```python
from build123d import *

# Parameters (mm, degrees)
BOSS_EXTRUDE1_DEPTH     = 32.5
SKETCH4_R               = 1.05
BOSS_EXTRUDE2_DEPTH     = 2.5
SKETCH5_R               = 1.05
BOSS_EXTRUDE3_DEPTH     = 3
CUT_EXTRUDE1_DEPTH      = 31.122
SKETCH13_W              = 30.122
SKETCH13_H              = 38
BOSS_EXTRUDE7_DEPTH     = 2.5
BOSS_EXTRUDE4_DEPTH     = 5
BOSS_EXTRUDE6_DEPTH     = 5
CUT_EXTRUDE2_DEPTH      = 6
SKETCH12_W              = 16.4999
SKETCH12_H              = 2
CUT_EXTRUDE4_DEPTH      = 10
CUT_EXTRUDE4_DEPTH_BACK = 23.5
CHAMFER1_SIZE           = 2
CHAMFER1_SIZE2          = 3.464101615


with BuildPart() as part:
    # Sketch2 → Boss-Extrude1 (new body)
    with BuildSketch(Plane(origin=(0, 0, 0), x_dir=(1, 0, 0), z_dir=(0, 1, 0))):
        Polygon((15.061, 0), (15.061, 32), (12.561, 32), (12.561, 2.5), (-12.561, 2.5), (-12.561, 32), (-15.061, 32), (-15.061, 0), align=None)
    extrude(amount=BOSS_EXTRUDE1_DEPTH)

    # Sketch4 → Boss-Extrude2 (add)
    with BuildSketch(Plane.XZ):
        Polygon((-7.5, -6), (7.5, -6), (12.561, -10), (15.061, -10), (15.061, 0), (-15.061, 0), (-15.061, -10), (-12.561, -10), align=None)
        with Locations((-10.2499, -4.95)):
            Circle(SKETCH4_R, mode=Mode.SUBTRACT)
        with Locations((10.2499, -4.95)):
            Circle(SKETCH4_R, mode=Mode.SUBTRACT)
    extrude(amount=BOSS_EXTRUDE2_DEPTH)

    # Sketch5 → Boss-Extrude3 (add)
    with BuildSketch(Plane(origin=(0, 32.5, 0), x_dir=(1, 0, 0), z_dir=(0, 1, 0))):
        Polygon((-15.061, 32), (-10.2499, 32), (-6.25, 26), (6.25, 26), (10.2499, 32), (15.061, 32), (15.061, 0), (-15.061, 0), align=None)
        with Locations((-10.2499, 8.7)):
            Circle(SKETCH5_R, mode=Mode.SUBTRACT)
        with Locations((10.2499, 8.7)):
            Circle(SKETCH5_R, mode=Mode.SUBTRACT)
    extrude(amount=BOSS_EXTRUDE3_DEPTH)

    # Sketch6 → Cut-Extrude1 (cut, through all)
    with BuildSketch(Plane.ZY.offset(15.061)):
        Polygon((-10, 0), (-32, 30.5), (-32, 0), align=None)
    extrude(amount=-CUT_EXTRUDE1_DEPTH, mode=Mode.SUBTRACT)

    # Sketch13 → Boss-Extrude7 (add)
    with BuildSketch(Plane.XY):
        with Locations((0, 16.5)):
            Rectangle(SKETCH13_W, SKETCH13_H)
    extrude(amount=BOSS_EXTRUDE7_DEPTH)

    # Sketch8 → Boss-Extrude4 (add)
    with BuildSketch(Plane.XY.offset(2.5)):
        Polygon((0, 76.5), (43.59255168, 16.5), (-43.59255168, 16.5), align=None)
    extrude(amount=BOSS_EXTRUDE4_DEPTH)

    # Sketch9 → Boss-Extrude6 (add)
    with BuildSketch(Plane.XY.offset(2.5)):
        Polygon((-43.59255168, 16.5), (-72.654252801, -23.5), (72.654252801, -23.5), (43.59255168, 16.5), align=None)
    extrude(amount=BOSS_EXTRUDE6_DEPTH)

    # Sketch10 → Cut-Extrude2 (cut, through all)
    with BuildSketch(Plane(origin=(0, 0, 2.5), x_dir=(-1, 0, 0), z_dir=(0, 0, -1))):
        Polygon((-43.59255168, -23.5), (-58.12340224, -3.5), (-72.654252801, -23.5), align=None)
        Polygon((72.654252801, -23.5), (58.12340224, -3.5), (43.59255168, -23.5), align=None)
    extrude(amount=-CUT_EXTRUDE2_DEPTH, mode=Mode.SUBTRACT)

    # Sketch12 → Cut-Extrude4 (cut, two sides)
    with BuildSketch(Plane(origin=(0, 0, -26), x_dir=(-1, 0, 0), z_dir=(0, 0, -1))) as cut_extrude4_sk:
        with Locations((0, 33.5)):
            Rectangle(SKETCH12_W, SKETCH12_H)
    extrude(amount=CUT_EXTRUDE4_DEPTH, mode=Mode.SUBTRACT)
    extrude(cut_extrude4_sk.sketch, amount=-CUT_EXTRUDE4_DEPTH_BACK, mode=Mode.SUBTRACT)

    # Chamfer1
    chamfer1_edges = [part.edges().sort_by_distance(p)[0] for p in [
        (-29.06170112, 36.5, 7.5),
        (0, -23.5, 7.5),
        (29.06170112, 36.5, 7.5),
        (50.85797696, -13.5, 7.5),
        (-50.85797696, -13.5, 7.5),
    ]]
    chamfer1_side = [part.faces().sort_by_distance(p)[0] for p in [
        (0, 12.152173913, 7.5),
    ]]
    chamfer(chamfer1_edges, length=CHAMFER1_SIZE, length2=CHAMFER1_SIZE2, reference=chamfer1_side[0])


solid = part.part
```
The model under review builds one solid part; all positions refer to its coordinate system, in mm. A direction names the side the tool comes from. Coordinates: 2 decimals unless noted, no trailing zeros. Write each loop counter-clockwise with the first axis right and the second up, starting at its lowest first coordinate (ties: lowest second). Pieces come first, ordered by that corner, then holes. Notation, with made-up numbers: (79.25, 39.25) - (130.25, 39.25) arc R23 cw to (130.25, 52.25) - close; hole circle Ø1 at (-28, 9.25). An arc over 180 degrees is marked (long way). Answer in a Markdown table with one row per item. Add a question column.
Q1. Consider section B-B on y = 11. Give the boundary of the cut face in (x, z).
Q2. Consider section C-C on z = -20. Give the boundary of the cut face in (x, y).
Q3. Consider section A-A on z = -27.5. Give the boundary of the cut face in (x, y), then the cut area to 3 significant figures.
Q4. Draft analysis for pull direction X (two halves, no side actions). For faces 4 (the face through (-50.96, -13.36, 3.26)), 5 (the face through (13.79, 15.04, -20.85)), 6 (the face through (12.561, 20, -14)), state which applies: +X half, -X half, draft (parallel to the pull), parting line (faces both ways), or undercut.
Q5. For faces 1 (the face through (-8.722, 34.312, -29.709)), 2 (the face through (0, 34.5, -16)), 3 (the face through (15.061, 20, -11)), list the 3-axis set-ups (+Z, -Z, +X, -X, +Y, -Y) from which the entire face can be reached by the end or side of a thin tool; tool diameter is ignored.
Q6. To check wall thickness, follow line 1 along X through (y, z) = (34.65, -8.7); line 2 along X through (y, z) = (14, -3.5); line 3 along X through (y, z) = (34, -8). State the ranges of each line that lie inside material, in increasing order. Write a range as from..to.
Q7. Consider section D-D on x = 40. Give the boundary of the cut face in (y, z).
Q8. Clearance check with flat-ended pins moving along their axes: pin 1 (1 mm diameter, centred on y = 33.5, z = -20.5, fed in from +X); pin 2 (1.2 mm diameter, centred on x = -14, y = -1, fed in from -Z); pin 3 (10 mm diameter, centred on y = 56.5, z = 1, fed in from -X). State where each tip first meets the part, or that it passes through.
Answers below:
| question | item | result |
|---|---|---|
| 1 | outline | (-47.59, 2.5) - (-15.06, 2.5) - (-15.06, -17.93) - (-12.56, -17.93) - (-12.56, -2.5) - (12.56, -2.5) - (12.56, -17.93) - (15.06, -17.93) - (15.06, 2.5) - (47.59, 2.5) - (47.59, 4.04) - (45.12, 7.5) - (-45.12, 7.5) - (-47.59, 4.04) - close |
| 2 | outline | (-15.06, 13.86) - (-12.56, 13.86) - (-12.56, 32.5) - (-8.25, 32.5) - (-8.25, 34.5) - (8.25, 34.5) - (8.25, 32.5) - (12.56, 32.5) - (12.56, 13.86) - (15.06, 13.86) - (15.06, 35.5) - (-15.06, 35.5) - close |
| 3 | outline | (-15.06, 24.26) - (-12.56, 24.26) - (-12.56, 32.5) - (-8.25, 32.5) - (-8.25, 34.5) - (-7.25, 34.5) - (-7.25, 35.5) - (-15.06, 35.5) - close; (7.25, 34.5) - (8.25, 34.5) - (8.25, 32.5) - (12.56, 32.5) - (12.56, 24.26) - (15.06, 24.26) - (15.06, 35.5) - (7.25, 35.5) - close |
| 3 | area | 84.1 mm² |
| 4 | face 4 | -X half |
| 4 | face 5 | draft |
| 4 | face 6 | undercut |
| 5 | face 1 | -Z, +Y, -Y |
| 5 | face 2 | -Z |
| 5 | face 3 | -Z, +X, +Y, -Y |
| 6 | line 1 | -15.06..-11.3, -9.2..9.2, 11.3..15.06 |
| 6 | line 2 | -15.06..-12.56, 12.56..15.06 |
| 6 | line 3 | -15.06..-11.03, -9.47..-8.25, 8.25..9.47, 11.03..15.06 |
| 7 | outline | (-23.5, 2.5) - (21.44, 2.5) - (21.44, 4.04) - (18.04, 7.5) - (-21.5, 7.5) - (-23.5, 4.04) - close |
| 8 | pin 1 | x = 15.06 |
| 8 | pin 2 | z = -10 |
| 8 | pin 3 | x = -18 |
